The model under review builds one solid part; all positions refer to its coordinate system, in mm. A direction names the side the tool comes from. Round coordinates to 2 decimals unless told otherwise and drop trailing zeros. Write each loop counter-clockwise with the first axis right and the second up, starting at its lowest first coordinate (ties: lowest second). Pieces come first, ordered by that corner, then holes. Notation, with made-up numbers: (73.5, 53.5) -> (90.5, 53.5) arc R29 ccw to (90.5, 77.5) -> close; hole circle Ø1 at (7, 88.25). An arc over 180 degrees is marked (long way). Answer as a JSON object with one key per item and string values. Group by question number.
1) We need section B-B, the plane y = 118.5. Write out the cut boundary in (x, z), then the cut area to 3 significant figures.
2) We need section C-C, the plane z = 8.75. Write out the cut boundary in (x, y).
3) We need section A-A, the plane x = -34. Write out the cut boundary in (y, z), then the cut area to 3 significant figures.
4) Mouldability with a two-part tool opening along X and no side actions: class faces 6 (the flat face through (-32, 135.408, 7)), 7 (the flat face through (-36, 135, 10)), 8 (the cylindrical face through (-44.84, 118.083, 13.496)) as pulls with the +X half, pulls with the -X half, needs draft (parallel to the pull), parting line crosses it, or undercut.
5) Insertion check: pin 1 Ø2 at (y, z) = (118, 11.5) entering from -X; pin 2 Ø2.5 at (x, z) = (-36.5, 6.5) entering from -Y; pin 3 Ø8 at (x, z) = (-43.5, 9) entering from +Y. Each pin has a flat end and moves straight along its axis. Give the tip position at first contact, or say it passes through.
6) Machinability: for faces 1 (the flat face through (-39.365, 120, 8)), 2 (the flat face through (-40, 135.408, 7)), 3 (the cylindrical face through (-44.84, 118.083, 1.504)), 4 (the flat face through (-36, 120, 10.6)), 5 (the flat face through (-36, 135.45, 8)), which of the approach directions +Z, -Z, +X, -X, +Y, -Y give a long, thin tool a straight path to every point of the face, cutting with its end or side? Answer none if there is none.
7) To check wall thickness, follow probe 1 along X at (y, z) = (129, 6); probe 2 along Y at (x, z) = (-39.25, 6); probe 3 along Z at (x, y) = (-36.5, 117). State the ranges of each line that lie inside material, in increasing order. Write a range as [from, to].
8) We need section D-D, the plane x = -42.75. Write out the cut boundary in (y, z), then the cut area to 3 significant figures.
from build123d import *

# Parameters (mm, degrees)
SKETCH1_W           = 20
SKETCH1_H           = 30
BOSS_EXTRUDE1_DEPTH = 15
SKETCH2_W           = 6.2
SKETCH2_H           = 6.2
CUT_EXTRUDE1_DEPTH  = 3.25
FILLET1_R           = 5
SKETCH4_W           = 6.2
SKETCH4_H           = 6.2
CUT_EXTRUDE2_DEPTH  = 68
SKETCH6_W           = 5
SKETCH6_H           = 1
BOSS_EXTRUDE3_DEPTH = 6.2


with BuildPart() as part:
    # Sketch1 → Boss-Extrude1 (new body)
    with BuildSketch(Plane.XY):
        with Locations((-36.265495527, 120.408164147)):
            Rectangle(SKETCH1_W, SKETCH1_H)
    extrude(amount=BOSS_EXTRUDE1_DEPTH)

    # Sketch2 → Cut-Extrude1 (cut)
    with BuildSketch(Plane(origin=(0, 105.408164147, 0), x_dir=(-1, 0, 0), z_dir=(0, -1, 0))):
        with Locations((36.265495527, -7.5)):
            Rectangle(SKETCH2_W, SKETCH2_H)
    extrude(amount=-CUT_EXTRUDE1_DEPTH, mode=Mode.SUBTRACT)

    # Fillet1
    fillet1_edges = [part.edges().sort_by_distance(p)[0] for p in [
        (-46.265495527, 120.408164147, 15),
        (-26.265495527, 120.408164147, 15),
        (-46.265495527, 120.408164147, 0),
        (-36.265495527, 135.408164147, 0),
        (-26.265495527, 120.408164147, 0),
        (-36.265495527, 135.408164147, 15),
        (-46.265495527, 135.408164147, 7.5),
        (-26.265495527, 135.408164147, 7.5),
    ]]
    fillet(fillet1_edges, radius=FILLET1_R)

    # Sketch4 → Cut-Extrude2 (cut)
    with BuildSketch(Plane.XZ.offset(-108.658164147)):
        with Locations((-36.265495527, 7.5)):
            Rectangle(SKETCH4_W, SKETCH4_H)
    extrude(amount=-CUT_EXTRUDE2_DEPTH, mode=Mode.SUBTRACT)

    # Sketch6 → Boss-Extrude3 (add)
    with BuildSketch(Plane(origin=(-39.365495527, 0, 0), x_dir=(0, 0, -1), z_dir=(1, 0, 0))):
        with Locations((-7.5, 134.949726458)):
            Rectangle(SKETCH6_W, SKETCH6_H)
    extrude(amount=BOSS_EXTRUDE3_DEPTH)


solid = part.part
Here are the results:
{
 "1": {"outline": "(-46.27, 5) arc R5 ccw to (-41.27, 0) -> (-31.27, 0) arc R5 ccw to (-26.27, 5) -> (-26.27, 10) arc R5 ccw to (-31.27, 15) -> (-41.27, 15) arc R5 ccw to (-46.27, 10) -> close; hole (-39.37, 4.4) -> (-33.17, 4.4) -> (-33.17, 10.6) -> (-39.37, 10.6) -> close", "area": "240 mm^2"},
 "2": {"outline": "(-46.27, 105.41) -> (-39.37, 105.41) -> (-39.37, 134.45) -> (-33.17, 134.45) -> (-33.17, 105.41) -> (-26.27, 105.41) -> (-26.27, 130.41) arc R5 ccw to (-31.27, 135.41) -> (-33.17, 135.41) -> (-33.17, 135.45) -> (-39.37, 135.45) -> (-39.37, 135.41) -> (-41.27, 135.41) arc R5 ccw to (-46.27, 130.41) -> close"},
 "3": {"outline": "(105.41, 0) -> (130.41, 0) arc R5 ccw to (135.37, 4.4) -> (105.41, 4.4) -> close; (105.41, 10.6) -> (135.37, 10.6) arc R5 ccw to (130.41, 15) -> (105.41, 15) -> close; (134.45, 5) -> (135.45, 5) -> (135.45, 10) -> (134.45, 10) -> close", "area": "258 mm^2"},
 "4": {"face 6": "needs draft", "face 7": "undercut", "face 8": "pulls with the -X half"},
 "5": {"pin 1": "stops at x = -46.24", "pin 2": "stops at y = 134.45", "pin 3": "stops at y = 135.41"},
 "6": {"face 1": "-Y", "face 2": "+Z, -Z, -X, +Y", "face 3": "-Z, -X, +Y, -Y", "face 4": "+Y, -Y", "face 5": "+Z, -Z, +X, -X, +Y"},
 "7": {"probe 1": "x = [-46.27, -39.37], [-33.17, -26.27]", "probe 2": "y = [134.45, 135.45]", "probe 3": "z = [0, 4.4], [10.6, 15]"},
 "8": {"outline": "(105.41, 0.23) -> (130.41, 0.23) arc R4.77 ccw to (135.18, 5) -> (135.18, 10) arc R4.77 ccw to (130.41, 14.77) -> (105.41, 14.77) -> close", "area": "423 mm^2"}
}
